Geometry check sheet. Reference: drawing and pictorial views, mm from the part's lowest x, y, z. Give positions to 0.01 mm unless a question says otherwise; leave off trailing zeros. Loops run counter-clockwise (first coordinate to the right, second up) from the corner with the lowest first, then second, coordinate; pieces in that order, holes last. Notation, with made-up numbers: M 46.5,56.25 L 105.5,56.25 A31 cw 105.5,92.25 Z; hole C -33.75,21.5 d4. An arc over 180 degrees is marked long. Put each result on its own line as item: value. Start each with the question number.
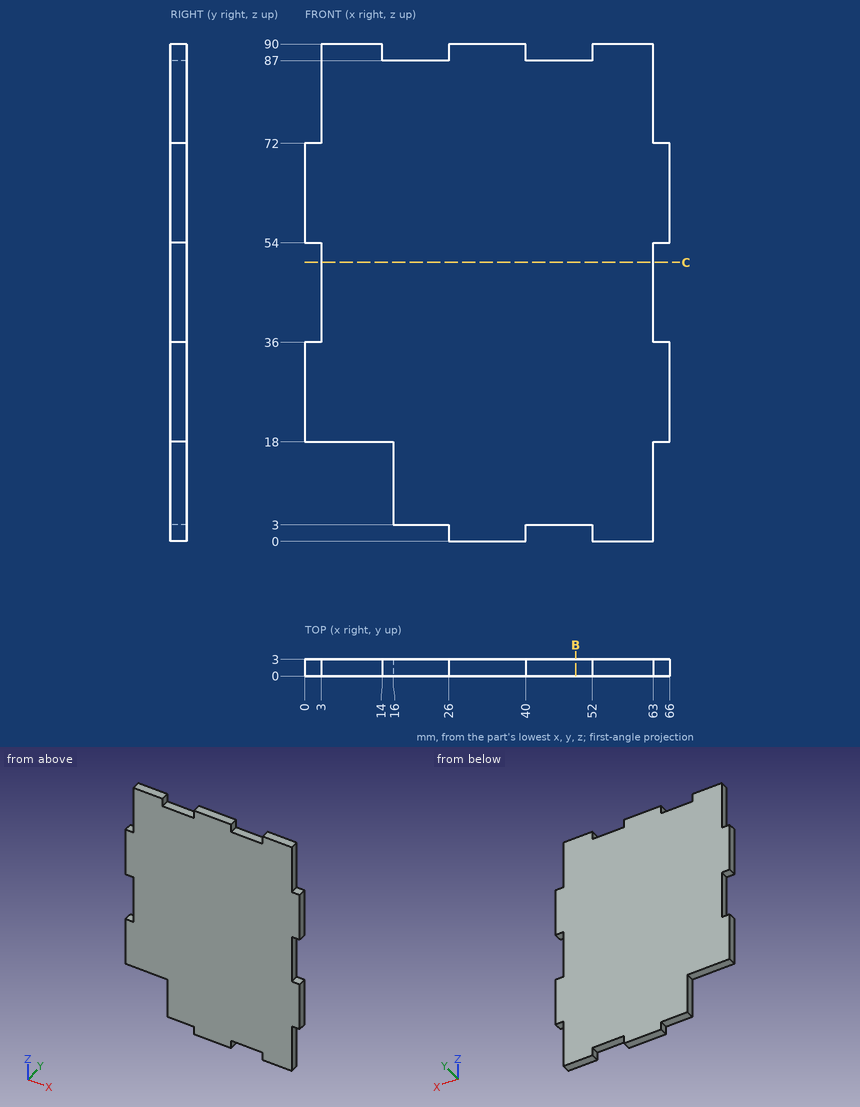
Q1. Section check B-B, the plane x = 49. Record the cut outline in (y, z).
Q2. Depth check by flat-ended pin: P1, Ø0.9, axis at x = 20.5, y = 2, coming from the +Z side; P2, Ø0.9, axis at x = 64.5, y = 1.5, coming from the -Z side; P3, Ø1.5, axis at y = 2, z = 43, coming from the -X side. Enter the tip coordinate at first touch or a pass-through.
Q3. Section check C-C, the plane z = 50.5. Record the cut outline in (x, y).
Q4. Thickness scan on line 1 along Z through (x, y) = (41, 1); line 2 along X through (y, z) = (1.9, 40.5); line 3 along Z through (x, y) = (6.5, 1.4). Record the ranges inside material, lowest first. Write a range as [from, to].
Found:
1. outline: M 0,3 L 3,3 L 3,87 L 0,87 Z
2. P1: stops at z = 87
2. P2: stops at z = 18
2. P3: stops at x = 3
3. outline: M 3,0 L 63,0 L 63,3 L 3,3 Z
4. line 1: z = [3, 87]
4. line 2: x = [3, 63]
4. line 3: z = [18, 90]
